Work out the finished part from the listing and answer in its coordinate system (mm). Face numbers are marked on the shaded views. A direction names the side the tool comes from. Coordinates: 2 decimals unless noted, no trailing zeros. Loops run counter-clockwise (first coordinate to the right, second up) from the corner with the lowest first, then second, coordinate; pieces in that order, holes last. Notation, with made-up numbers: (68.5, 67.25) -> (97.5, 67.25) arc R16 cw to (97.5, 73.25) -> close; hole circle Ø9 at (-36.75, 1.5). An arc over 180 degrees is marked (long way). One line per question, with ' | ' between items.
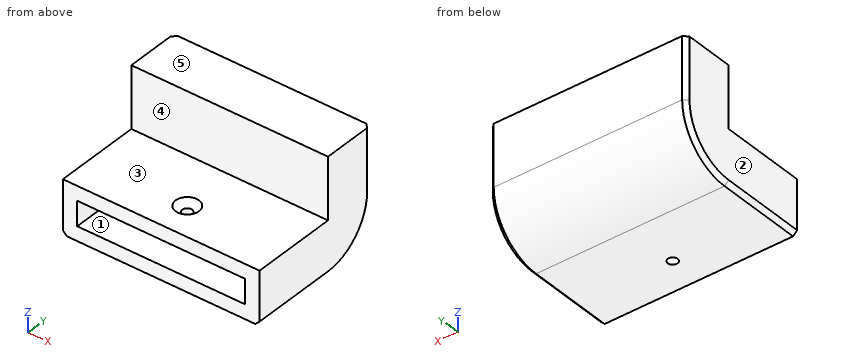
```python
from build123d import *

# Parameters (mm, degrees)
SKETCH1_W           = 60.96
SKETCH1_H           = 16.51
SKETCH1_W_2         = 50.8
SKETCH1_H_2         = 6.35
BOSS_EXTRUDE1_DEPTH = 19.05
BOSS_EXTRUDE2_DEPTH = 60.96
SKETCH6_W           = 60.96
SKETCH6_H           = 16.51
SKETCH6_W_2         = 50.8
SKETCH6_H_2         = 6.35
BOSS_EXTRUDE3_DEPTH = 7.62
SKETCH7_W           = 50.8
SKETCH7_H           = 6.35
BOSS_EXTRUDE4_DEPTH = 7.62
SKETCH9_R           = 1.524
CUT_EXTRUDE1_DEPTH  = 51.561314263
CHAMFER1_SIZE       = 2.1082
CHAMFER1_SIZE2      = 1.832630301
SKETCH11_W          = 52.07
SKETCH11_H          = 7.62
CUT_EXTRUDE2_DEPTH  = 19.05
CHAMFER2_SIZE       = 1.27


with BuildPart() as part:
    # Sketch1 → Boss-Extrude1 (new body)
    with BuildSketch(Plane(origin=(0, 0, 0), x_dir=(1, 0, 0), z_dir=(0, 1, 0))):
        Rectangle(SKETCH1_W, SKETCH1_H)
        Rectangle(SKETCH1_W_2, SKETCH1_H_2, mode=Mode.SUBTRACT)
    extrude(amount=BOSS_EXTRUDE1_DEPTH)

    # Sketch5 → Boss-Extrude2 (add)
    with BuildSketch(Plane(origin=(30.48, 0, 0), x_dir=(0, 0, -1), z_dir=(1, 0, 0))):
        with BuildLine():
            Line((-8.255, 35.56), (-27.305, 35.56))
            Line((-27.305, 35.56), (-27.305, 19.05))
            Line((-27.305, 19.05), (-8.255, 19.05))
            Line((-8.255, 19.05), (8.255, 19.05))
            ThreePointArc((8.255, 19.05), (3.419332957, 30.724332957), (-8.255, 35.56))
        make_face()
    extrude(amount=-BOSS_EXTRUDE2_DEPTH)

    # Sketch6 → Boss-Extrude3 (add)
    with BuildSketch(Plane.XZ):
        Rectangle(SKETCH6_W, SKETCH6_H)
        Rectangle(SKETCH6_W_2, SKETCH6_H_2, mode=Mode.SUBTRACT)
    extrude(amount=BOSS_EXTRUDE3_DEPTH)

    # Sketch7 → Boss-Extrude4 (add)
    with BuildSketch(Plane.XZ.offset(-19.05)):
        Rectangle(SKETCH7_W, SKETCH7_H)
    extrude(amount=BOSS_EXTRUDE4_DEPTH)

    # Sketch9 → Cut-Extrude1 (cut, through all)
    with BuildSketch(Plane.XY.offset(8.255)):
        with Locations((0, 2.54)):
            Circle(SKETCH9_R)
    extrude(amount=-CUT_EXTRUDE1_DEPTH, mode=Mode.SUBTRACT)

    # Chamfer1
    chamfer1_edges = [part.edges().sort_by_distance(p)[0] for p in [
        (-1.524, 2.54, 8.255),
    ]]
    chamfer1_side = [part.faces().sort_by_distance(p)[0] for p in [
        (0, 5.729313606, 8.255),
    ]]
    chamfer(chamfer1_edges, length=CHAMFER1_SIZE, length2=CHAMFER1_SIZE2, reference=chamfer1_side[0])

    # Sketch11 → Cut-Extrude2 (cut)
    with BuildSketch(Plane.XZ.offset(7.62)):
        Rectangle(SKETCH11_W, SKETCH11_H)
    extrude(amount=-CUT_EXTRUDE2_DEPTH, mode=Mode.SUBTRACT)

    # Chamfer2
    chamfer2_edges = [part.edges().sort_by_distance(p)[0] for p in [
        (30.48, 30.724332957, -3.419332957),
        (30.48, 35.56, 17.78),
        (-30.48, 30.724332957, -3.419332957),
        (-30.48, 35.56, 17.78),
        (-30.48, 5.715, -8.255),
        (30.48, 5.715, -8.255),
    ]]
    chamfer(chamfer2_edges, length=CHAMFER2_SIZE)


solid = part.part
```
1) Find section B-B (y = 2.54). Write down the section's boundary in (x, z) (3 decimals), plus the area to 3 significant figures.
Check values:
outline: (-30.48, -6.985) -> (-29.21, -8.255) -> (-1.524, -8.255) -> (-1.524, -3.81) -> (-26.035, -3.81) -> (-26.035, 3.81) -> (-1.524, 3.81) -> (-1.524, 6.422) -> (-3.632, 8.255) -> (-30.48, 8.255) -> close; (1.524, -8.255) -> (29.21, -8.255) -> (30.48, -6.985) -> (30.48, 8.255) -> (3.632, 8.255) -> (1.524, 6.422) -> (1.524, 3.81) -> (26.035, 3.81) -> (26.035, -3.81) -> (1.524, -3.81) -> close | area: 577 mm^2
2) For the marked faces 4 and 5, determine the directions among +Z, -Z, +X, -X, +Y, -Y from which every point of the face is accessible in a straight line to the end or side of a thin tool.
Check values:
face 4: +Z, +X, -X, -Y | face 5: +Z, +X, -X, +Y, -Y
3) The mould has two halves that part along X. Classify the marked faces 1, 2 and 3: released by +X, released by -X, zero draft, split by the parting line, or undercut.
Check values:
face 1: undercut | face 2: released by -X | face 3: zero draft
4) Find the intervals of material crossed by line 1 along Z through (x, y) = (14.5, 3.5) (3 decimals); line 2 along Z through (x, y) = (7.5, 18.5) (3 decimals); line 3 along Y through (x, z) = (0, -6.95), in increasing order.
Check values:
line 1: z = -8.255 to -3.81, 3.81 to 8.255 | line 2: z = -8.255 to 8.255 | line 3: y = -7.62 to 1.02, 4.06 to 25.48
5) Flat-ended cylindrical pins translate along their axes: pin 1 (5 mm diameter, centred on x = 0, y = 2.54, fed in from +Z); pin 2 (9.5 mm diameter, centred on x = 2, y = -0.5, fed in from +Z) (3 decimals); pin 3 (6 mm diameter, centred on x = 4.5, z = 0.5, fed in from -Y). Find the tip coordinate at first contact, or state that the pin passes through.
Check values:
pin 1: stops at z = 7.27 | pin 2: stops at z = 8.255 | pin 3: stops at y = 11.43
6) Find section C-C (y = -4). Write down the section's boundary in (x, z) (3 decimals), plus the area to 3 significant figures.
Check values:
outline: (-30.48, -6.985) -> (-29.21, -8.255) -> (29.21, -8.255) -> (30.48, -6.985) -> (30.48, 8.255) -> (-30.48, 8.255) -> close; hole (-26.035, -3.81) -> (26.035, -3.81) -> (26.035, 3.81) -> (-26.035, 3.81) -> close | area: 608 mm^2
7) Find section D-D (x = 19). Write down the section's boundary in (y, z) (3 decimals), plus the area to 3 significant figures.
Check values:
outline: (-7.62, -8.255) -> (19.05, -8.255) arc R16.51 ccw to (35.56, 8.255) -> (35.56, 27.305) -> (19.05, 27.305) -> (19.05, 8.255) -> (-7.62, 8.255) -> (-7.62, 3.81) -> (11.43, 3.81) -> (11.43, -3.81) -> (-7.62, -3.81) -> close | area: 824 mm^2
8) Find section A-A (x = 0). Write down the section's boundary in (y, z) (3 decimals), plus the area to 3 significant figures.
Check values:
outline: (-7.62, -8.255) -> (1.016, -8.255) -> (1.016, -3.81) -> (-7.62, -3.81) -> close; (-7.62, 3.81) -> (1.016, 3.81) -> (1.016, 6.422) -> (-1.092, 8.255) -> (-7.62, 8.255) -> close; (4.064, -8.255) -> (19.05, -8.255) arc R16.51 ccw to (35.56, 8.255) -> (35.56, 27.305) -> (19.05, 27.305) -> (19.05, 8.255) -> (6.172, 8.255) -> (4.064, 6.422) -> (4.064, 3.81) -> (11.43, 3.81) -> (11.43, -3.81) -> (4.064, -3.81) -> close | area: 793 mm^2
